from build123d import *

# Parameters (mm, degrees)
ESQUISSE2_W             = 95.7
ESQUISSE2_H             = 95.7
BOSS_EXTRU_1_DEPTH      = 59.2
ESQUISSE3_R             = 16
BOSS_EXTRU_2_DEPTH      = 13.2
ESQUISSE4_W             = 78.5
ESQUISSE4_H             = 78.5
ESQUISSE4_R             = 17.15
ESQUISSE4_R_2           = 9.75
ENL_V_MAT_EXTRU_1_DEPTH = 51.1


with BuildPart() as part:
    # Esquisse2 → Boss.-Extru.1 (new body)
    with BuildSketch(Plane.XY):
        with Locations((47.85, 47.85)):
            Rectangle(ESQUISSE2_W, ESQUISSE2_H)
    extrude(amount=BOSS_EXTRU_1_DEPTH)

    # Esquisse3 → Boss.-Extru.2 (add)
    with BuildSketch(Plane.XY.offset(59.2)):
        with Locations(Location((23.925, 71.775, 0), (0, 0, 180))):
            Circle(ESQUISSE3_R)
        with Locations(Location((71.775, 71.775, 0), (0, 0, 180))):
            Circle(ESQUISSE3_R)
        with Locations(Location((71.775, 23.925, 0), (0, 0, 180))):
            Circle(ESQUISSE3_R)
        with Locations(Location((23.925, 23.925, 0), (0, 0, 180))):
            Circle(ESQUISSE3_R)
    extrude(amount=BOSS_EXTRU_2_DEPTH)

    # Esquisse4 → Enlèv. mat.-Extru.1 (cut)
    # profile 1 of 2: a face of its own
    with BuildSketch(Plane(origin=(0, 0, 0), x_dir=(-1, 0, 0), z_dir=(0, 0, -1))):
        with Locations((-47.85, 47.85)):
            Rectangle(ESQUISSE4_W, ESQUISSE4_H)
        with Locations((-47.85, 47.85)):
            Circle(ESQUISSE4_R, mode=Mode.SUBTRACT)
    # profile 2 of 2: a face of its own
    with BuildSketch(Plane(origin=(0, 0, 0), x_dir=(-1, 0, 0), z_dir=(0, 0, -1))):
        with Locations((-47.85, 47.85)):
            Circle(ESQUISSE4_R_2)
    extrude(amount=-ENL_V_MAT_EXTRU_1_DEPTH, mode=Mode.SUBTRACT)


solid = part.part
Here's how the part is built. I have some questions about the finished solid (model axes, mm). A direction names the side the tool comes from. Coordinates: 2 decimals unless noted, no trailing zeros. Write each loop counter-clockwise with the first axis right and the second up, starting at its lowest first coordinate (ties: lowest second). Pieces come first, ordered by that corner, then holes.
Item 1: If I drill on line 1 (Y direction, x = 24.5, z = 33.5); line 2 (Y direction, x = 47.85, z = 39); line 3 (X direction, y = 45, z = 37.5), over which ranges is the centre line in solid material (lowest first)?
Item 2: On a 3-axis mill with a long thin cutter (end or side, diameter ignored), from which of +Z, -Z, +X, -X, +Y, -Y can I reach the whole of each face in a straight line? I mean faces 1 (the cylindrical face through (8.664, 66.969, 65.708)), 2 (the flat face through (55, 40, 0)), 3 (the cylindrical face through (32, 41.3, 25.2)). Say none if no direction works.
Item 3: I want a section at B-B on y = 47.85. Write out the boundary of the cut face in (x, z).
Item 4: Will these pins go through, and if not, where does the flat tip stop? pin 1 (4 mm diameter, centred on y = 66, z = 64.5, fed in from -X); pin 2 (6 mm diameter, centred on x = 52.5, y = 47, fed in from -Z); pin 3 (6 mm diameter, centred on x = 56, y = 40.5, fed in from +Z).
Item 5: If we mould it in two halves opening along Y, with no side actions, what happens to faces 4 (the flat face through (47, 95.7, 29)), 5 (the flat face through (72, 24, 72.4)), 6 (the flat face through (87.1, 47, 25)), 7 (the flat face through (47, 0, 29))? For each: +Y half, -Y half, draft (parallel to the pull), parting line (faces both ways), or undercut.
Item 6: I want a section at D-D on y = 60. Write out the boundary of the cut face in (x, z).
Item 7: I want a section at A-A on z = 29. Write out the boundary of the cut face in (x, y).
Findings below:
1. line 1: y = 0 to 8.6, 87.1 to 95.7
1. line 2: y = 0 to 8.6, 30.7 to 38.1, 57.6 to 65, 87.1 to 95.7
1. line 3: x = 0 to 8.6, 30.94 to 38.53, 57.17 to 64.76, 87.1 to 95.7
2. face 1: +Z
2. face 2: -Z, +X, -X, +Y, -Y
2. face 3: -Z
3. outline: (0, 0) - (8.6, 0) - (8.6, 51.1) - (30.7, 51.1) - (30.7, 0) - (38.1, 0) - (38.1, 51.1) - (57.6, 51.1) - (57.6, 0) - (65, 0) - (65, 51.1) - (87.1, 51.1) - (87.1, 0) - (95.7, 0) - (95.7, 59.2) - (0, 59.2) - close
4. pin 1: stops at x = 8.38
4. pin 2: stops at z = 51.1
4. pin 3: stops at z = 59.2
5. face 4: +Y half
5. face 5: draft
5. face 6: undercut
5. face 7: -Y half
6. outline: (0, 0) - (8.6, 0) - (8.6, 51.1) - (35.75, 51.1) - (35.75, 0) - (59.95, 0) - (59.95, 51.1) - (87.1, 51.1) - (87.1, 0) - (95.7, 0) - (95.7, 59.2) - (82.61, 59.2) - (82.61, 72.4) - (60.94, 72.4) - (60.94, 59.2) - (34.76, 59.2) - (34.76, 72.4) - (13.09, 72.4) - (13.09, 59.2) - (0, 59.2) - close
7. outline: (0, 0) - (95.7, 0) - (95.7, 95.7) - (0, 95.7) - close; circle Ø34.3 at (47.85, 47.85); hole (8.6, 8.6) - (87.1, 8.6) - (87.1, 87.1) - (8.6, 87.1) - close; hole circle Ø19.5 at (47.85, 47.85)
